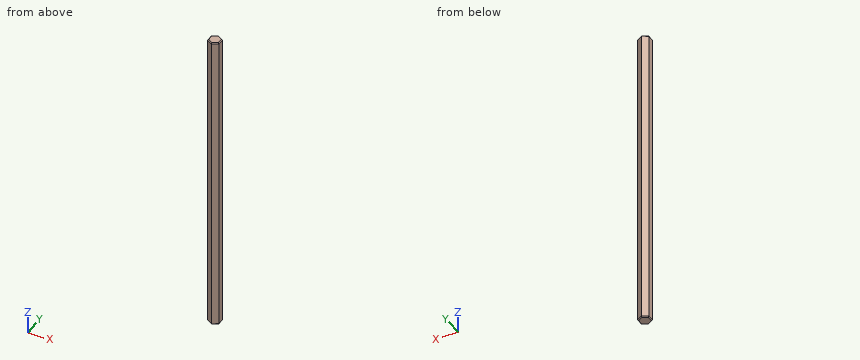
from build123d import *

# Parameters (mm, degrees)
BOSS_EXTRUDE1_DEPTH = 135
CHAMFER1_SIZE       = 0.4


with BuildPart() as part:
    # Sketch1 → Boss-Extrude1 (new body)
    with BuildSketch(Plane.XY.offset(67.5)):
        Polygon((0, -2.886751346), (2.5, -1.443375673), (2.5, 1.443375673), (0, 2.886751346), (-2.5, 1.443375673), (-2.5, -1.443375673), align=None)
    extrude(amount=-BOSS_EXTRUDE1_DEPTH)

    # Chamfer1
    chamfer1_edges = [part.edges().sort_by_distance(p)[0] for p in [
        (2.5, 0, -67.5),
        (1.25, 2.165063509, -67.5),
        (-1.25, 2.165063509, -67.5),
        (-2.5, 0, -67.5),
        (-1.25, -2.165063509, -67.5),
        (-2.5, 0, 67.5),
        (-1.25, 2.165063509, 67.5),
        (1.25, 2.165063509, 67.5),
        (1.25, -2.165063509, -67.5),
        (2.5, 0, 67.5),
        (1.25, -2.165063509, 67.5),
        (-1.25, -2.165063509, 67.5),
    ]]
    chamfer(chamfer1_edges, length=CHAMFER1_SIZE)


solid = part.part
The model under review builds one solid part; all positions refer to its coordinate system, in mm. Give positions to 0.01 mm unless a question says otherwise; leave off trailing zeros. Write each loop counter-clockwise with the first axis right and the second up, starting at its lowest first coordinate (ties: lowest second). Pieces come first, ordered by that corner, then holes.
1. Add section A-A, the plane x = -1.3. Write out the cut boundary in (y, z), plus the area to 3 significant figures.
2. Wall thickness on L1, parallel to X at y = -1.45, z = -3; L2, parallel to Y at x = 1.35, z = 56; L3, parallel to Y at x = -1.55, z = 2.5: over which ranges is each line inside the solid? List them lowest first.
3. Add section B-B, the plane z = -12. Write out the cut boundary in (x, y).
Worked answers:
1. outline: (-2.14, -67.1) - (-1.67, -67.5) - (1.67, -67.5) - (2.14, -67.1) - (2.14, 67.1) - (1.67, 67.5) - (-1.67, 67.5) - (-2.14, 67.1) - close
1. area: 576 mm2
2. L1: x = -2.49 to 2.49
2. L2: y = -2.11 to 2.11
2. L3: y = -1.99 to 1.99
3. outline: (-2.5, -1.44) - (0, -2.89) - (2.5, -1.44) - (2.5, 1.44) - (0, 2.89) - (-2.5, 1.44) - close
